Autodesk Fusion 360 part; units mm, degrees
sketch "Skizze1" plane through (0, 0, 0) normal (0, 1, 0) x (1, 0, 0)
  circle A0 centre (0.1472, 12.45) radius 1.6
  circle A1 centre (0.1472, -12.45) radius 1.6
  line L0 (0, 0) -> (50, 0) construction
  line L1 (4.1472, 12.45) -> (4.1472, -12.45)
  line L2 (-3.8528, 12.45) -> (-3.8528, -12.45)
  arc A2 (4.1472, 12.45) -> (-3.8528, 12.45) centre (0.1472, 12.45) ccw
  arc A3 (-3.8528, -12.45) -> (4.1472, -12.45) centre (0.1472, -12.45) ccw
  dimension "d1" = 24.9
  dimension "d2" = 3.2
  dimension "d3" = 8
extrude "Extrusion1" add sketch "Skizze1" along normal blind 3
sketch "Skizze2" plane through (4.1472, 0, 0) normal (1, 0, 0) x (0, 0, -1)
  line L0 (-12.45, 0) -> (12.45, 0)
  line L1 (12.45, 0) -> (12.45, 3)
  line L2 (12.45, 3) -> (-12.45, 3)
  line L3 (-12.45, 3) -> (-12.45, 0)
  arc A0 (3.2, 35) -> (-3.1577, 35.5188) centre (0, 35) ccw
  line L4 (0, 0) -> (0, 43) construction
  circle A1 centre (0, 35) radius 1.6
  circle A2 centre (0, 15) radius 1.6
  line L5 (0, 25) -> (20, 25) construction
  line L6 (8.5, 3) -> (3.2, 17)
  line L7 (3.2, 17) -> (3.2, 35)
  line L8 (-3.1577, 35.5188) -> (-8.5, 3)
  dimension "d7" = 25
  dimension "d8" = 3.2
  dimension "d9" = 20
  dimension "d10" = 3.2
  dimension "d17" = 8.5
  dimension "d18" = 14
  dimension "d19" = 8.5
extrude "Extrusion2" add sketch "Skizze2" against normal blind 8 contours L2 A0 L6 L7 L8
fillet "Abrundung3" radius 1 3 edges at (0.1472, 17, -3.2) (0.1472, 3, -8.5) (0.1472, 3, 8.5)
Design review of the part built by this model. Coordinates are the model's own, in mm. A direction names the side the tool comes from. Round coordinates to 2 decimals unless told otherwise and drop trailing zeros. Order: outer loops, then holes, each group sorted by start corner. A loop starts at its lowest first (then second) coordinate and runs counter-clockwise, first axis right, second up.
1) For L1, parallel to Y at x = 1, z = 0; L2, parallel to Y at x = 0.25, z = -0.5; L3, parallel to Y at x = -1.75, z = 13.5, list the stretches that pass through material, from the lowest coordinate up.
The answers:
L1: y = 0 to 13.4, 16.6 to 33.4, 36.6 to 38.2
L2: y = 0 to 13.48, 16.52 to 33.48, 36.52 to 38.16
L3: y = 0 to 3
2) Clearance check with flat-ended pins moving along their axes: pin 1 Ø2 at (x, z) = (2, -12) entering from +Y; pin 2 Ø2 at (x, z) = (-2, -13) entering from -Y; pin 3 Ø4 at (x, y) = (0, 25) entering from +Z; pin 4 Ø2.5 at (x, y) = (-1.5, 23) entering from -Z. State where each tip first meets the part, or that it passes through.
The answers:
pin 1: stops at y = 3
pin 2: stops at y = 0
pin 3: stops at z = 5.21
pin 4: stops at z = -3.2
3) Consider section D-D (x = -2.5). State the section outline as (y, z) points, plus the area to 3 significant figures.
The answers:
outline: (0, -15.45) - (3, -15.45) - (3, -9.19) arc R1 cw to (3.65, -8.26) - (16.83, -3.26) arc R1 cw to (17.18, -3.2) - (35, -3.2) arc R3.2 ccw to (35.52, 3.16) - (3.84, 8.36) arc R1 cw to (3, 9.35) - (3, 15.45) - (0, 15.45) - close; hole circle Ø3.2 at (15, 0); hole circle Ø3.2 at (35, 0)
area: 420 mm2
4) Draft analysis for pull direction X (two halves, no side actions). For faces 1 (the flat face through (0.203, 19.9, 5.724)), 2 (the flat face through (-3.853, 15, 3)), 3 (the cylindrical face through (-0.2, 1.48, 10.89)), state which applies: released by +X, released by -X, zero draft, split by the parting line, or undercut.
The answers:
face 1: zero draft
face 2: released by -X
face 3: undercut
5) Consider section A-A (z = 0). State the section outline as (x, y) points, plus the area to 3 significant figures.
The answers:
outline: (-3.85, 0) - (4.15, 0) - (4.15, 13.4) - (-3.85, 13.4) - close; (-3.85, 16.6) - (4.15, 16.6) - (4.15, 33.4) - (-3.85, 33.4) - close; (-3.85, 36.6) - (4.15, 36.6) - (4.15, 38.2) - (-3.85, 38.2) - close
area: 254 mm2
6) Consider section B-B (x = -0.25). State the section outline as (y, z) points.
The answers:
outline: (0, -16.43) - (3, -16.43) - (3, -14) - (0, -14) - close; (0, -10.9) - (3, -10.9) - (3, -9.19) arc R1 cw to (3.65, -8.26) - (16.83, -3.26) arc R1 cw to (17.18, -3.2) - (35, -3.2) arc R3.2 ccw to (35.52, 3.16) - (3.84, 8.36) arc R1 cw to (3, 9.35) - (3, 10.9) - (0, 10.9) - close; (0, 14) - (3, 14) - (3, 16.43) - (0, 16.43) - close; hole circle Ø3.2 at (15, 0); hole circle Ø3.2 at (35, 0)
7) Machinability: for faces 4 (the flat face through (-2, 3, -13)), 5 (the cylindrical face through (0.203, 38.183, -0.327)), 6 (the flat face through (2, 3, 13)), which of the approach directions +Z, -Z, +X, -X, +Y, -Y give a long, thin tool a straight path to every point of the face, cutting with its end or side? Answer none if there is none.
The answers:
face 4: -Z, +X, -X, +Y
face 5: +X, -X, +Y
face 6: +Z, +X, -X, +Y
8) Consider section C-C (y = 16). State the section outline as (x, z) points.
The answers:
outline: (-3.85, -3.58) - (4.15, -3.58) - (4.15, -1.25) - (-3.85, -1.25) - close; (-3.85, 1.25) - (4.15, 1.25) - (4.15, 6.36) - (-3.85, 6.36) - close
